Could you check a few things on this model? Use its own coordinates, in mm. A direction names the side the tool comes from. Give positions to 0.01 mm unless a question says otherwise; leave off trailing zeros. Order: outer loops, then holes, each group sorted by start corner. A loop starts at its lowest first (then second) coordinate and runs counter-clockwise, first axis right, second up.
from build123d import *

# Parameters (mm, degrees)
SKETCH1_R           = 50
BOSS_EXTRUDE1_DEPTH = 23
SKETCH2_R           = 3.96875
CUT_EXTRUDE1_DEPTH  = 23
BOSS_EXTRUDE2_START = -2
SKETCH3_R           = 50
SKETCH3_R_2         = 45.5
BOSS_EXTRUDE2_DEPTH = 2
CUT_EXTRUDE2_DEPTH  = 108.888625907
FILLET1_R           = 4.953
SKETCH6_R           = 3.175
CUT_EXTRUDE4_DEPTH  = 30.48
BOSS_EXTRUDE4_DEPTH = 23
FILLET2_R           = 12.7
SKETCH9_W           = 23
SKETCH9_H           = 150.8
SKETCH9_R           = 3.96875
BOSS_EXTRUDE5_DEPTH = 25.4


with BuildPart() as part:
    # Sketch1 → Boss-Extrude1 (new body)
    with BuildSketch(Plane.XY):
        with BuildLine():
            Line((73.66, 75.4), (73.66, -75.4))
            Line((73.66, -75.4), (60.96, -75.4))
            Line((60.96, -75.4), (60.96, -59.525))
            ThreePointArc((60.96, -59.525), (60.03006403, -57.27993597), (57.785, -56.35))
            Line((57.785, -56.35), (0, -56.35))
            ThreePointArc((0, -56.35), (-56.35, 0), (0, 56.35))
            Line((0, 56.35), (57.785, 56.35))
            ThreePointArc((57.785, 56.35), (60.03006403, 57.27993597), (60.96, 59.525))
            Line((60.96, 59.525), (60.96, 75.4))
            Line((60.96, 75.4), (73.66, 75.4))
        make_face()
        Circle(SKETCH1_R, mode=Mode.SUBTRACT)
    extrude(amount=-BOSS_EXTRUDE1_DEPTH)

    # Sketch2 → Cut-Extrude1 (cut)
    with BuildSketch(Plane.ZY.offset(-60.96)):
        with Locations((-11.5, 67.4625)):
            Circle(SKETCH2_R)
        with Locations((-11.5, -67.4625)):
            Circle(SKETCH2_R)
    extrude(amount=-CUT_EXTRUDE1_DEPTH, mode=Mode.SUBTRACT)

    # Sketch3 → Boss-Extrude2 (add)
    with BuildSketch(Plane(origin=(0, 0, -23), x_dir=(-1, 0, 0), z_dir=(0, 0, -1)).offset(BOSS_EXTRUDE2_START)):
        with Locations(Location((0, 0, 0), (0, 0, 180))):
            Circle(SKETCH3_R)
        Circle(SKETCH3_R_2, mode=Mode.SUBTRACT)
    extrude(amount=BOSS_EXTRUDE2_DEPTH)

    # Sketch4 → Cut-Extrude2 (cut, through all)
    with BuildSketch(Plane.XY):
        with BuildLine():
            Line((64.77, 8.89), (64.77, 47.46))
            Line((64.77, 47.46), (30.355226425, 47.46))
            ThreePointArc((30.355226425, 47.46), (47.120470693, 30.879647228), (55.631459367, 8.89))
            Line((55.631459367, 8.89), (64.77, 8.89))
        make_face()
        with BuildLine():
            Line((30.355226425, -47.46), (64.77, -47.46))
            Line((64.77, -47.46), (64.77, -8.89))
            Line((64.77, -8.89), (55.631459367, -8.89))
            ThreePointArc((55.631459367, -8.89), (47.120470693, -30.879647228), (30.355226425, -47.46))
        make_face()
    extrude(amount=-CUT_EXTRUDE2_DEPTH, mode=Mode.SUBTRACT)

    # Fillet1
    fillet1_edges = [part.edges().sort_by_distance(p)[0] for p in [
        (30.355226425, -47.46, -11.5),
        (55.631459367, -8.89, -11.5),
        (64.77, -8.89, -11.5),
        (64.77, -47.46, -11.5),
        (55.631459367, 8.89, -11.5),
        (30.355226425, 47.46, -11.5),
        (64.77, 47.46, -11.5),
        (64.77, 8.89, -11.5),
    ]]
    fillet(fillet1_edges, radius=FILLET1_R)

    # Sketch6 → Cut-Extrude4 (cut)
    with BuildSketch(Plane.XY):
        with Locations((-27.94, -50)):
            Circle(SKETCH6_R)
        with Locations((29.21, -50)):
            Circle(SKETCH6_R)
    extrude(amount=-CUT_EXTRUDE4_DEPTH, mode=Mode.SUBTRACT)

    # Sketch8 → Boss-Extrude4 (add)
    with BuildSketch(Plane.XY):
        with BuildLine():
            Line((-39.555189909, -40.133644879), (-35.840291724, -52.393828665))
            ThreePointArc((-35.840291724, -52.393828665), (-32.642189928, -56.784868082), (-27.407882123, -58.23783197))
            Line((-27.407882123, -58.23783197), (3.632324942, -56.232808177))
            ThreePointArc((3.632324942, -56.232808177), (-10.963276805, -55.273221922), (-24.82017584, -50.58934049))
            ThreePointArc((-24.82017584, -50.58934049), (-29.488783115, -52.771623326), (-30.076991341, -47.651831989))
            ThreePointArc((-30.076991341, -47.651831989), (-35.018437298, -44.147837424), (-39.555189909, -40.133644879))
        make_face()
    extrude(amount=-BOSS_EXTRUDE4_DEPTH)

    # Fillet2
    fillet2_edges = [part.edges().sort_by_distance(p)[0] for p in [
        (-39.555189909, -40.133644879, -11.5),
    ]]
    fillet(fillet2_edges, radius=FILLET2_R)

    # Sketch9 → Boss-Extrude5 (add)
    with BuildSketch(Plane(origin=(73.66, 0, 0), x_dir=(0, 0, -1), z_dir=(1, 0, 0))):
        with Locations((11.5, 0)):
            Rectangle(SKETCH9_W, SKETCH9_H)
        with Locations(Location((11.5, 67.4625, 0), (0, 0, 180))):
            Circle(SKETCH9_R, mode=Mode.SUBTRACT)
        with Locations(Location((11.5, -67.4625, 0), (0, 0, 180))):
            Circle(SKETCH9_R, mode=Mode.SUBTRACT)
    extrude(amount=BOSS_EXTRUDE5_DEPTH)


solid = part.part
Item 1: For pin 1 (1.5 mm diameter, centred on x = -5, z = -13, fed in from +Y); pin 2 (12 mm diameter, centred on x = -26, z = -7.5, fed in from +Y); pin 3 (7 mm diameter, centred on x = 18.5, z = -15, fed in from -Y); pin 4 (10.5 mm diameter, centred on y = -67.46, z = -11.5, fed in from +X), each with a flat end and sliding along its axis, tell me the tip position at first contact or that it passes through.
Findings:
pin 1: stops at y = 56.19
pin 2: stops at y = 52.68
pin 3: stops at y = -56.35
pin 4: stops at x = 99.06
Item 2: Imagine slicing it at B-B on y = -27. List the corners of the cut face in (x, z) for me, then the cut area to 3 significant figures.
Findings:
outline: (-49.46, -23) - (-36.62, -23) - (-36.62, -21) - (-42.08, -21) - (-42.08, 0) - (-49.46, 0) - close; (36.62, -23) - (49.45, -23) - (49.45, 0) - (42.08, 0) - (42.08, -21) - (36.62, -21) - close; (64.77, -23) - (99.06, -23) - (99.06, 0) - (64.77, 0) - close
area: 1,150 mm2
Item 3: We'd pull the mould along X, two halves only. Please class faces 1 (the cylindrical face through (-51.96, 21.81, -11.34)), 2 (the cylindrical face through (36.107, -27.686, -21.986)), 3 (the flat face through (22, 41, -21)), 4 (the flat face through (28, 56.35, -11)): +X half, -X half, draft (parallel to the pull), parting line (faces both ways), or undercut.
Findings:
face 1: -X half
face 2: undercut
face 3: undercut
face 4: draft
Item 4: Imagine slicing it at A-A on x = 29.21. List the corners of the cut face in (y, z) for me (3 decimals), then the cut area to 3 significant figures.
Findings:
outline: (-56.35, -23) - (-53.175, -23) - (-53.175, 0) - (-56.35, 0) - close; (-46.825, -23) - (-34.886, -23) - (-34.886, -21) - (-40.58, -21) - (-40.58, 0) - (-46.825, 0) - close; (34.886, -23) - (56.35, -23) - (56.35, 0) - (40.58, 0) - (40.58, -21) - (34.886, -21) - close
area: 602 mm2
Item 5: Please list where these lines run through material, in increasing order: line 1 along Y through (x, z) = (83, -11.5); line 2 along Y through (x, z) = (85, -8.25); line 3 along X through (y, z) = (-15, -9).
Findings:
line 1: y = -75.4 to -71.43, -63.49 to 63.49, 71.43 to 75.4
line 2: y = -75.4 to -69.74, -65.18 to 65.18, 69.74 to 75.4
line 3: x = -54.32 to -47.7, 47.7 to 54.3, 64.77 to 99.06
Item 6: For faces 5 (the flat face through (60.96, 71, -9)), 6 (the flat face through (30, -56.35, -11)), 7 (the flat face through (60.96, -71, -14)), 8 (the cylindrical face through (63.28, -46.05, -11.66)), 9 (the cylindrical face through (79.743, 71.337, -12.36)), which set-ups out of +Z, -Z, +X, -X, +Y, -Y let a thin tool reach every point of the face, with its end or its side?
Findings:
face 5: +Z, -Z, -X, +Y
face 6: +Z, -Z, -Y
face 7: +Z, -Z, -X, -Y
face 8: +Z, -Z
face 9: +X, -X
Item 7: Imagine slicing it at C-C on z = -2.5. Give the number of separate pieces and of enclosed holes in the cut face, then the cut area to 3 significant figures.
Findings:
separate pieces: 1
enclosed holes: 5
area: 8,610 mm2
